from build123d import *

# Parameters (mm, degrees)
SKETCH1_R           = 28.5
SKETCH1_R_2         = 21
BOSS_EXTRUDE1_DEPTH = 13.175
SKETCH2_R           = 2.25
CUT_EXTRUDE1_DEPTH  = 43.403780787
CIRPATTERN1_COUNT   = 4


with BuildPart() as part:
    # Sketch1 → Boss-Extrude1 (new, symmetric)
    with BuildSketch(Plane(origin=(0, 0, 0), x_dir=(1, 0, 0), z_dir=(0, 1, 0))):
        with Locations(Location((0, 0, 0), (0, 0, 90))):
            Circle(SKETCH1_R)
        with Locations(Location((0, 0, 0), (0, 0, 90))):
            Circle(SKETCH1_R_2, mode=Mode.SUBTRACT)
    extrude(amount=BOSS_EXTRUDE1_DEPTH, both=True)

    # Sketch2 → Cut-Extrude1 (cut, through all)
    with BuildSketch(Plane.XY):
        with Locations(Location((0, 8.175, 0), (0, 0, 90))):
            Circle(SKETCH2_R)
        with Locations(Location((0, -8.175, 0), (0, 0, 90))):
            Circle(SKETCH2_R)
    cut_extrude1 = extrude(amount=-CUT_EXTRUDE1_DEPTH, mode=Mode.SUBTRACT)

    # CirPattern1: Cut-Extrude1 ×4 about axis
    cirpattern1_axis = Axis((0, 13.175, 0), (0, -1, 0))
    for i in range(1, CIRPATTERN1_COUNT):
        add(cut_extrude1.rotate(cirpattern1_axis, i * 360 / CIRPATTERN1_COUNT), mode=Mode.SUBTRACT)


solid = part.part
Verification items for the finished model (mm, model axes). Round coordinates to 2 decimals unless told otherwise and drop trailing zeros. Write each loop counter-clockwise with the first axis right and the second up, starting at its lowest first coordinate (ties: lowest second). Pieces come first, ordered by that corner, then holes.
(1) Mould release check, pull along X, two halves, no side actions. Record for faces 1 (the cylindrical face through (-24.64, 10.32, 0.68)), 2 (the cylindrical face through (10.916, 0.184, -26.327)), 3 (the cylindrical face through (-0.68, -6.03, -24.64)): pulls with the +X half, pulls with the -X half, needs draft (parallel to the pull), parting line crosses it, or undercut.
Returned:
face 1: needs draft
face 2: parting line crosses it
face 3: undercut
(2) Section check C-C (x = 7). Enter the section's corners in (y, z) (3 decimals).
Returned:
outline: (-13.175, -27.627) - (13.175, -27.627) - (13.175, -19.799) - (-13.175, -19.799) - close; (-13.175, 19.799) - (13.175, 19.799) - (13.175, 27.627) - (-13.175, 27.627) - close
(3) Section check B-B (x = 0). Enter the section's corners in (y, z) (3 decimals), plus the area to 3 significant figures.
Returned:
outline: (-13.175, -28.5) - (-10.425, -28.5) - (-10.425, -21) - (-13.175, -21) - close; (-13.175, 21) - (-10.425, 21) - (-10.425, 28.5) - (-13.175, 28.5) - close; (-5.925, -28.5) - (5.925, -28.5) - (5.925, -21) - (-5.925, -21) - close; (-5.925, 21) - (5.925, 21) - (5.925, 28.5) - (-5.925, 28.5) - close; (10.425, -28.5) - (13.175, -28.5) - (13.175, -21) - (10.425, -21) - close; (10.425, 21) - (13.175, 21) - (13.175, 28.5) - (10.425, 28.5) - close
area: 260 mm2
(4) Section check A-A (z = 0). Enter the section's corners in (x, y) (3 decimals).
Returned:
outline: (-28.5, -13.175) - (-21, -13.175) - (-21, -10.425) - (-28.5, -10.425) - close; (-28.5, -5.925) - (-21, -5.925) - (-21, 5.925) - (-28.5, 5.925) - close; (-28.5, 10.425) - (-21, 10.425) - (-21, 13.175) - (-28.5, 13.175) - close; (21, -13.175) - (28.5, -13.175) - (28.5, -10.425) - (21, -10.425) - close; (21, -5.925) - (28.5, -5.925) - (28.5, 5.925) - (21, 5.925) - close; (21, 10.425) - (28.5, 10.425) - (28.5, 13.175) - (21, 13.175) - close
(5) Depth check by flat-ended pin: pin 1 Ø1.5 at (x, y) = (10, 3) entering from -Z; pin 2 Ø8 at (x, y) = (12, 5.5) entering from -Z; pin 3 Ø3 at (x, y) = (22, 5) entering from +Z; pin 4 Ø4 at (y, z) = (8.175, 0) entering from -X. Enter the tip coordinate at first touch or a pass-through.
Returned:
pin 1: stops at z = -26.96
pin 2: stops at z = -27.35
pin 3: stops at z = 19.8
pin 4: passes through
(6) Material ranges on line 1 (Y direction, x = 24.5, z = 0) (3 decimals); line 2 (Y direction, x = -2, z = -22.5) (3 decimals); line 3 (X direction, y = 10, z = -16), recorded low to high.
Returned:
line 1: y = -13.175 to -10.425, -5.925 to 5.925, 10.425 to 13.175
line 2: y = -13.175 to -9.206, -7.144 to 7.144, 9.206 to 13.175
line 3: x = -23.58 to -13.6, 13.6 to 23.58
(7) Section check D-D (z = 8). Enter the section's corners in (x, y) (3 decimals), plus the area to 3 significant figures.
Returned:
outline: (-27.354, -13.175) - (-19.416, -13.175) - (-19.416, 13.175) - (-27.354, 13.175) - close; (19.416, -13.175) - (27.354, -13.175) - (27.354, 13.175) - (19.416, 13.175) - close
area: 418 mm2
